The model under review builds one solid part; all positions refer to its coordinate system, in mm. A direction names the side the tool comes from. Coordinates: 2 decimals unless noted, no trailing zeros. Order: outer loops, then holes, each group sorted by start corner. A loop starts at its lowest first (then second) coordinate and runs counter-clockwise, first axis right, second up.
Autodesk Inventor part; units mm, degrees
ref_plane "Work Plane1" through (0, 5, 0) normal (0, 1, 0) x (-1, 0, 0)
ref_plane "YZ Plane" through (0, 0, 0) normal (1, 0, 0) x (0, 1, 0)
ref_plane "XY Plane" through (0, 0, 0) normal (0, 0, 1) x (1, 0, 0)
sketch "Sketch1" plane through (0, 0, 0) normal (0, 1, 0) x (-1, 0, 0)
  circle A0 centre (0, 0) radius 1.5
  circle A1 centre (0, 0) radius 3
  circle A2 centre (-58, 0) radius 1.5
  circle A3 centre (-58, 0) radius 3
  circle A4 centre (0, -49) radius 1.375
  circle A5 centre (0, -49) radius 3
  circle A6 centre (-58, -49) radius 1.375
  circle A7 centre (-58, -49) radius 3
  dimension "d0" = 3
  dimension "d1" = 6
  dimension "d2" = 3
  dimension "d3" = 6
  dimension "d4" = 58
  dimension "d5" = 2.75
  dimension "d6" = 6
  dimension "d9" = 49
  dimension "d10" = 2.75
  dimension "d11" = 6
extrude "Extrusion1" add sketch "Sketch1" along normal blind 10
ref_plane "Work Plane1" through (0, 5, 0) normal (0, 1, 0) x (-1, 0, 0)
sketch "Sketch2" plane through (0, 5, 0) normal (0, 1, 0) x (-1, 0, 0)
  circle A0 centre (0, -49) radius 3
  circle A1 centre (0, 0) radius 3
  circle A2 centre (-58, 0) radius 3
  circle A3 centre (-58, -49) radius 3
  circle A4 centre (0, -49) radius 3
  circle A5 centre (0, 0) radius 3
  circle A6 centre (-58, -49) radius 3
  circle A7 centre (0, -49) radius 1.375
  circle A8 centre (-58, 0) radius 1.5
  line L0 (3, -49) -> (3, 0)
  line L1 (0, -52) -> (-58, -52)
  line L2 (-61, -49) -> (-61, 0)
  circle A9 centre (-58, 0) radius 3
  line L3 (-58, 3) -> (0, 3)
  line L4 (-3, -49) -> (-3, 0)
  line L5 (0, -46) -> (-58, -46)
  line L6 (-55, -49) -> (-55, 0)
  line L7 (-58, -3) -> (0, -3)
  line L8 (-55, -47) -> (-3, -47)
  line L9 (-55, -41) -> (-3, -41)
  line L10 (-55, -8) -> (-3, -8)
  line L11 (-55, -2) -> (-3, -2)
  line L12 (0, -46) -> (10, -46)
  line L13 (10, -46) -> (10, -41)
  line L14 (10, -41) -> (-3, -41)
  line L15 (-3, -8) -> (10, -8)
  line L16 (10, -8) -> (10, -3)
  line L17 (0, -3) -> (10, -3)
  line L18 (10, -41) -> (10, -8)
  line L19 (5, -41) -> (5, -8)
  line L20 (-24, -46) -> (-24, -8)
  line L21 (-29, -46) -> (-29, -8)
  point P0 (-3, -46)
  point P1 (-55, -46)
  point P2 (-55, -3)
  point P3 (-3, -3)
  point P4 (3, 0)
  point P5 (0, 3)
  point P6 (-61, 0)
  point P7 (-44, -3)
  point P8 (-39, -3)
  point P9 (3, -3)
  point P10 (3, -8)
  point P11 (-24, -41)
  point P12 (-29, -41)
  dimension "d23" = -1
  dimension "d25" = -1
  dimension "d45" = 39
  dimension "d46" = 10
  dimension "d47" = 5
  dimension "d48" = 34
  dimension "d49" = 5
  dimension "d77" = 5
  dimension "d78" = 5
extrude "Extrusion2" add sketch "Sketch2" along normal up to surface (5 mm away) contours A0 L12 L0 | A0 L4 L5 | L5 L4 L14 L0 L12 | L1 A3 L6 L8 L4 A0 | L0 L14 L13 L12 | L5 L20 L9 L4 | L14 L4 L15 L0 | L5 L21 L9 L20 | L2 A2 L7 L6 L5 A3 | A3 L5 L6 | L15 L4 L7 L17 L0 | L0 L17 L16 L15 | L19 L15 L18 L14 | L10 L6 L7 L4 | L9 L21 L10 L20 | L5 L6 L9 L21 | L17 A1 L0 | L4 A1 L7 | L3 A1 L4 L11 L6 A2 | A2 L6 L7
sketch "Sketch8" plane through (-10, 5, -3) normal (0, 0, 1) x (1, 0, 0)
  line L0 (7, 5) -> (0, 5)
  line L1 (10, 5) -> (7, 5)
  line L2 (68, 5) -> (10, 5)
  line L3 (71, 5) -> (68, 5)
  line L4 (39, 0) -> (39, 5)
  line L5 (39, 5) -> (39, 10)
  line L6 (39, 10) -> (71, 5)
  line L7 (0, 5) -> (7, 5)
  line L8 (0, 5) -> (0, 10)
  line L9 (0, 10) -> (39, 10)
  point P0 (10, -5)
  dimension "d50" = 5
  dimension "d51" = 5
extrude "Extrusion8" add sketch "Sketch8" against normal up to surface (5 mm away)
sketch "Sketch9" plane through (-3, 5, -46) normal (0, 0, -1) x (-1, 0, 0)
  line L0 (-32, 10) -> (7, 10)
  line L1 (-64, 5) -> (-32, 10)
  line L2 (-58, 5) -> (-64, 5)
  line L3 (-3, 5) -> (-61, 5)
  line L4 (0, 5) -> (-3, 5)
  line L5 (7, 5) -> (0, 5)
  line L6 (7, 10) -> (7, 5)
  point P0 (-3, -5)
extrude "Extrusion9" add sketch "Sketch9" against normal up to surface (5 mm away)
sketch "Sketch10" plane through (-10, 5, -46) normal (-1, 0, 0) x (0, 0, 1)
  line L0 (38, 5) -> (5, 5)
  line L1 (5, 5) -> (5, 10)
  line L2 (0, 10) -> (5, 10)
  line L3 (0, 0) -> (0, 10)
  line L4 (0, 0) -> (43, 0)
  line L5 (43, 0) -> (43, 10)
  line L6 (43, 10) -> (38, 10)
  line L7 (38, 10) -> (38, 5)
  line L8 (0, 10) -> (5, 10)
  line L9 (5, 10) -> (38, 10)
  point P0 (46, -5)
extrude "Extrusion10" add sketch "Sketch10" against normal up to surface (5 mm away) contours L0 L1 L9 L7
sketch "Sketch11" plane through (29, 5, -8) normal (1, 0, 0) x (0, 0, -1)
  line L0 (0, 10) -> (33, 10)
  line L1 (33, 5) -> (0, 5)
  line L2 (0, 0) -> (0, 10)
  line L3 (33, 0) -> (33, 10)
  point P0 (-8, -5)
extrude "Extrusion11" add sketch "Sketch11" against normal up to surface (5 mm away)
sketch "Sketch12" plane through (-10, 15, -3) normal (0, 1, 0) x (1, 0, 0)
  circle A0 centre (2.5, 2) radius 1.5
  circle A1 centre (2.5, 41) radius 1.5
  line L0 (0, 43) -> (0, 0)
  line L1 (39, 0) -> (0, 0)
  line L2 (0, 43) -> (39, 43)
  circle A2 centre (36.5, 2) radius 1.5
  circle A3 centre (36.5, 41) radius 1.5
  line L3 (39, 38) -> (39, 5)
  line L4 (5, 38) -> (34, 38)
  line L5 (34, 5) -> (5, 5)
  point P0 (10, -3)
  dimension "d60" = 3
  dimension "d61" = 3
  dimension "d62" = 2.5
  dimension "d64" = 2.5
  dimension "d66" = 3
  dimension "d67" = 3
  dimension "d69" = 2.5
  dimension "d70" = 2.5
  dimension "d79" = 39
  dimension "d80" = 39
  dimension "d81" = 3
  dimension "d82" = 3
  dimension "d83" = 3
  dimension "d84" = 3
extrude "Extrusion12" cut sketch "Sketch12" against normal up to surface (10 mm away)
sketch "Sketch13" plane through (-10, 5, -46) normal (-1, 0, 0) x (0, 0, 1)
  line L0 (5, 0) -> (5, 10)
  line L1 (38, 0) -> (38, 10)
  line L2 (0, 10) -> (43, 10)
  line L3 (0, 0) -> (43, 0)
  point P0 (46, -5)
extrude "Extrusion13" cut sketch "Sketch13" against normal blind 5
sketch "Sketch14" plane through (55, 5, -46) normal (0, 0, -1) x (-1, 0, 0)
  line L0 (0, 0) -> (0, 5)
  line L1 (0, 0) -> (52, 0)
  line L2 (52, 0) -> (52, 5)
  line L3 (58, 5) -> (52, 5)
  line L4 (58, 0) -> (58, 5)
  line L5 (58, 0) -> (65, 0)
  line L6 (65, 0) -> (65, 10)
  line L7 (65, 10) -> (26, 10)
  line L8 (26, 10) -> (-6, 5)
  line L9 (0, 5) -> (-6, 5)
  point P0 (55, -5)
extrude "Extrusion14" add sketch "Sketch14" along normal up to surface (1 mm away)
sketch "Sketch15" plane through (3, 5, -3) normal (0, 0, 1) x (1, 0, 0)
  line L0 (0, 0) -> (0, 5)
  line L1 (0, 0) -> (52, 0)
  line L2 (52, 0) -> (52, 5)
  line L3 (58, 5) -> (52, 5)
  line L4 (58, 5) -> (26, 10)
  line L5 (26, 10) -> (-13, 10)
  line L6 (-13, 0) -> (-13, 10)
  line L7 (-13, 0) -> (-6, 0)
  line L8 (-6, 0) -> (-6, 5)
  line L9 (0, 5) -> (-6, 5)
  point P0 (-3, -5)
extrude "Extrusion15" add sketch "Sketch15" along normal up to surface (1 mm away)
sketch "Sketch16" plane through (0, 10, 0) normal (0, 1, 0) x (1, 0, 0)
  circle A0 centre (0, 0) radius 1.5
  circle A1 centre (0, 0) radius 3
  circle A2 centre (0, 49) radius 1.375
  circle A3 centre (0, 49) radius 3
  circle A4 centre (58, 49) radius 1.375
  circle A5 centre (58, 49) radius 3
  circle A6 centre (58, 0) radius 1.5
  circle A7 centre (58, 0) radius 3
extrude "Extrusion16" cut sketch "Sketch16" along normal up to surface (5 mm away)
equation "\"d2\" = d0"
equation "\"d3\" = d1"
equation "\"d5\" = d7"
equation "\"d6\" = d8"
equation "\"d10\" = d12"
equation "\"d11\" = d13"
equation "\"d23\" = d25"
equation "\"d47\" = d21"
equation "\"d49\" = d21"
equation "\"d51\" = d50"
equation "\"d61\" = d60"
equation "\"d66\" = d60"
equation "\"d67\" = d60"
equation "\"d80\" = d79"
equation "\"d81\" = d82"
equation "\"d83\" = d82"
properties part number "Houder_RPI_v2"
(1) Wall thickness on probe 1 along X at (y, z) = (5.25, 0); probe 2 along X at (y, z) = (3.25, 0); probe 3 along X at (y, z) = (8.25, -49) (3 decimals): over which ranges is each line inside the solid? List them lowest first.
A:
probe 1: x = -3 to -1.5, 1.5 to 56.5, 59.5 to 61
probe 2: x = -3 to -1.5, 1.5 to 3, 55 to 56.5, 59.5 to 61
probe 3: x = -3 to -1.375, 1.375 to 56.625, 59.375 to 61
(2) We need section C-C, the plane y = 6. Count the separate pieces of the cut face and the enclosed holes in it, and give its area (3 significant figures).
A:
separate pieces: 1
enclosed holes: 10
area: 1,990 mm2
(3) Machinability: for faces 1 (the face through (23, 12, -2)), 2 (the face through (29, 10, -24)), 3 (the face through (-3, 7, -1)), 4 (the face through (25, 5, -25)), which of the approach directions +Z, -Z, +X, -X, +Y, -Y give a long, thin tool a straight path to every point of the face, cutting with its end or side? Answer none if there is none.
A:
face 1: +Z, +X, -X, +Y
face 2: +Y, -Y
face 3: +Z, -X, +Y, -Y
face 4: -Y
(4) We need section D-D, the plane y = 13.75. Write out the cut boundary in (x, z).
A:
outline: (-10, -47) - (-2.24, -47) arc R3 cw to (2.24, -47) - (37, -47) - (37, -41) - (29, -41) - (29, -8) - (37, -8) - (37, -2) - (2.24, -2) arc R3 cw to (-2.24, -2) - (-10, -2) - (-10, -8) - (24, -8) - (24, -41) - (-10, -41) - close; hole circle Ø3 at (-7.5, -44); hole circle Ø3 at (-7.5, -5); hole circle Ø3 at (26.5, -44); hole circle Ø3 at (26.5, -5)
(5) For pin 1 Ø2.5 at (x, z) = (-7.5, -5) entering from -Y (3 decimals); pin 2 Ø5 at (x, z) = (-7.5, -44) entering from -Y; pin 3 Ø3 at (y, z) = (11, -24) entering from +X; pin 4 Ø2 at (y, z) = (8, -0.5) entering from -X, all flat-tipped, find the tip position at first contact; note any pin that passes through.
A:
pin 1: passes through
pin 2: stops at y = 5
pin 3: stops at x = 61
pin 4: stops at x = -3
(6) We need section A-A, the plane z = -44. Write out the cut boundary in (x, y), and give its area (3 significant figures).
A:
outline: (-10, 5) - (-9, 5) - (-9, 15) - (-10, 15) - close; (-6, 5) - (25, 5) - (25, 15) - (-6, 15) - close; (28, 5) - (61, 5) - (61, 10) - (29, 15) - (28, 15) - close
area: 570 mm2
(7) Draft analysis for pull direction X (two halves, no side actions). For faces 5 (the face through (44.776, 12.535, -43.958)), 6 (the face through (-3, 7, -48)), 7 (the face through (-1.61, 3.82, -51.53)), state which applies: released by +X, released by -X, zero draft, split by the parting line, or undercut.
A:
face 5: released by +X
face 6: released by -X
face 7: undercut
(8) We need section B-B, the plane x = 26.5. Write out the cut boundary in (y, z).
A:
outline: (5, -52) - (10, -52) - (10, -47) - (15, -47) - (15, -45.5) - (5, -45.5) - close; (5, -42.5) - (15, -42.5) - (15, -6.5) - (5, -6.5) - close; (5, -3.5) - (15, -3.5) - (15, -2) - (10, -2) - (10, 3) - (5, 3) - close
